```python
from build123d import *

# Parameters (mm, degrees)
SKETCH2_W           = 213.36
SKETCH2_H           = 213.36
SKETCH2_R           = 93.98
BOSS_EXTRUDE1_DEPTH = 50.8
SKETCH4_W           = 431.498092941
SKETCH4_H           = 427.351859682
CUT_EXTRUDE1_DEPTH  = 106.68
FILLET1_R           = 2.54


with BuildPart() as part:
    # Sketch2 → Boss-Extrude1 (new body)
    with BuildSketch(Plane.XY.offset(50.8)):
        Rectangle(SKETCH2_W, SKETCH2_H)
        Circle(SKETCH2_R, mode=Mode.SUBTRACT)
    extrude(amount=-BOSS_EXTRUDE1_DEPTH)

    # Cut-Loft1: read off the stored shape, not the designer's step
    # Cut-Loft1: loft between two sections, ruled curve by curve
    cut_loft1_from = [
        Edge.make_bspline([(-5.225836659, 98.922061398, 0), (-203.069959455, 88.47038808, 0), (-192.618286137, -109.373734716, 0), (5.225836659, -98.922061398, 0), (203.069959455, -88.47038808, 0), (192.618286137, 109.373734716, 0), (-5.225836659, 98.922061398, 0)], [0, 0, 0, 0, 0.5, 0.5, 0.5, 1, 1, 1, 1], 3, [1, 0.333333333, 0.333333333, 1, 0.333333333, 0.333333333, 1]),
    ]
    cut_loft1_to = [
        Edge.make_bspline([(82.069205503, 45.791766816, 50.8), (-9.514328128, 209.930177822, 50.8), (-173.652739134, 118.34664419, 50.8), (-82.069205503, -45.791766816, 50.8), (9.514328128, -209.930177822, 50.8), (173.652739134, -118.34664419, 50.8), (82.069205503, 45.791766816, 50.8)], [0, 0, 0, 0, 0.5, 0.5, 0.5, 1, 1, 1, 1], 3, [1, 0.333333333, 0.333333333, 1, 0.333333333, 0.333333333, 1]),
    ]
    cut_loft1 = Solid(Shell([*[Face.make_surface_from_curves(cut_loft1_from[k], cut_loft1_to[k]) for k in range(1)], Face(Wire(cut_loft1_from)), Face(Wire(cut_loft1_to))]))
    add(cut_loft1, mode=Mode.SUBTRACT)

    # Sketch4 → Cut-Extrude1 (cut)
    with BuildSketch(Plane(origin=(0, 106.68, 0), x_dir=(1, 0, 0), z_dir=(0, 1, 0))):
        with Locations((-43.743226098, -53.764043901)):
            Rectangle(SKETCH4_W, SKETCH4_H)
    extrude(amount=-CUT_EXTRUDE1_DEPTH, mode=Mode.SUBTRACT)

    # Fillet1
    fillet1_edges = [part.edges().sort_by_distance(p)[0] for p in [
        (93.98, 0, 27.785112978),
        (-93.98, 0, 27.785112678),
    ]]
    fillet(fillet1_edges, radius=FILLET1_R)


solid = part.part
```
Source: CAD feature listing. Evaluate the final solid. Frame: model axes, mm. Give positions to 0.01 mm unless a question says otherwise; leave off trailing zeros. Loops run counter-clockwise (first coordinate to the right, second up) from the corner with the lowest first, then second, coordinate; pieces in that order, holes last. Notation, with made-up numbers: (20, 25.5) - (77, 25.5) arc R25 ccw to (77, 37.5) - close; hole circle Ø11 at (15, 83). An arc over 180 degrees is marked (long way). Use CSV: the item, a comma, the result in double quotes. Start each with the question number.
1. Section A-A (z = 38.5). Output: boundary loops of the cut face in (x, y), then the cut area to 3 significant figures.
2. Ray query, L1, parallel to X at y = -20.5, z = 8.5; L2, parallel to X at y = -60.5, z = 29.5; L3, parallel to Y at x = -8.5, z = 29.5. Return the intervals inside material, ascending.
3. Pin query (flat end, axial travel): pin 1 (1 mm diameter, centred on x = 64.5, z = 17.5, fed in from +Y); pin 2 (6 mm diameter, centred on x = -13, z = 17, fed in from +Y); pin 3 (6 mm diameter, centred on x = -71.5, y = -82.5, fed in from -Z). Return the tip coordinate at first contact, or that it passes through.
4. Draft query along X for faces 1 (the flat face through (-106.68, -54, 26)), 2 (the flat face through (7, -101, 0)), 3 (the flat face through (106.68, -54, 26)), 4 (the cylindrical face through (-2.03, -93.96, 28.11)). Return one class per face: +X half, -X half, draft (parallel to the pull), parting line (faces both ways), or undercut.
Response:
1,outline,"(-106.68, -106.68) - (106.68, -106.68) - (106.68, 0) - (96.49, 0) arc R2.54 ccw to (93.95, -2.47) arc R93.98 cw to (-93.95, -2.47) arc R2.54 ccw to (-96.49, 0) - (-106.68, 0) - close"
1,area,"8,880 mm²"
2,L1,"-106.68 to -91.72, 91.72 to 106.68"
2,L2,"-106.68 to -71.92, 71.92 to 106.68"
2,L3,"-106.68 to -93.59"
3,pin 1,"y = -67.88"
3,pin 2,"y = -92.61"
3,pin 3,"z = 0"
4,face 1,"-X half"
4,face 2,"draft"
4,face 3,"+X half"
4,face 4,"undercut"
